Could you check a few things on this drawing? It's one solid part, dimensions in mm from its lowest x, y, z. A direction names the side the tool comes from. Round coordinates to 2 decimals unless told otherwise and drop trailing zeros. Loops run counter-clockwise (first coordinate to the right, second up) from the corner with the lowest first, then second, coordinate; pieces in that order, holes last. Notation, with made-up numbers: (29, 83.5) -> (88, 83.5) arc R34 cw to (88, 121.5) -> close; hole circle Ø10 at (56.5, -13). An arc over 180 degrees is marked (long way). Write each question's results on one line, items separated by ' | '.
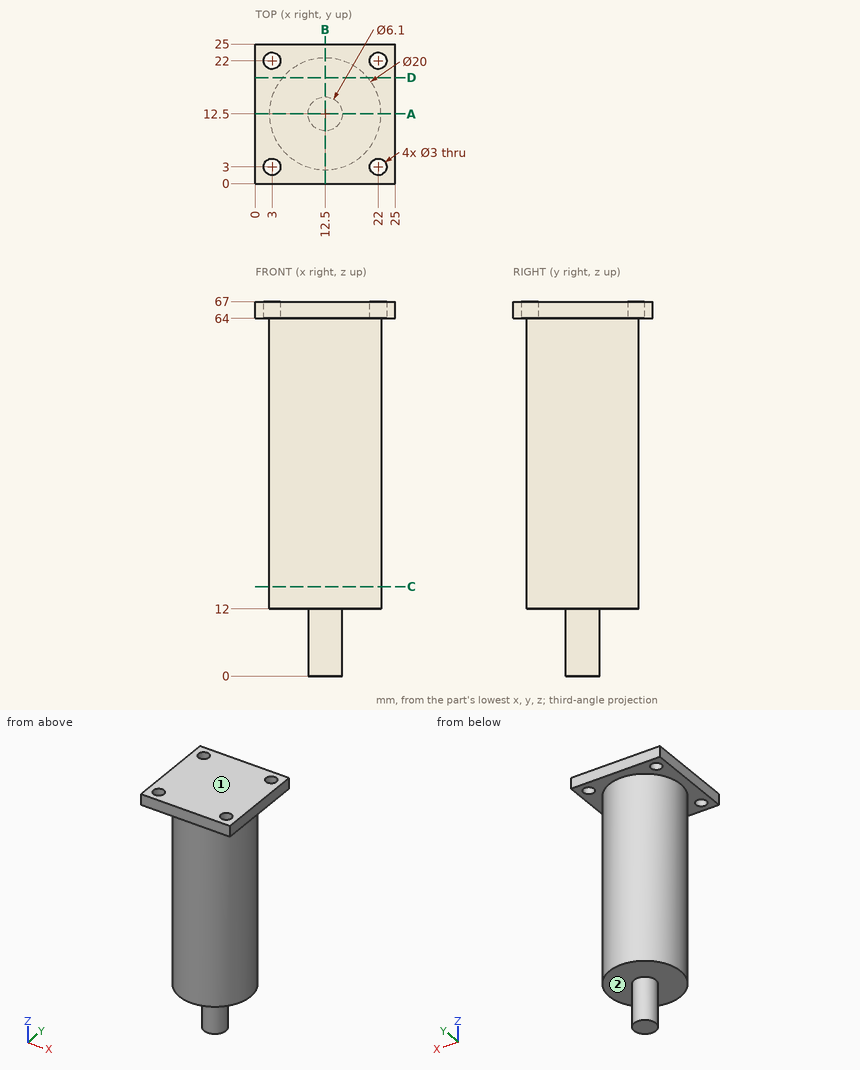
1) I want a section at D-D, the plane y = 19. Write out the boundary of the cut face in (x, z).
Model answer:
outline: (0, 64) -> (4.9, 64) -> (4.9, 12) -> (20.1, 12) -> (20.1, 64) -> (25, 64) -> (25, 67) -> (0, 67) -> close
2) I want a section at A-A, the plane y = 12.5. Write out the boundary of the cut face in (x, z), plus the area to 3 significant figures.
Model answer:
outline: (0, 64) -> (2.5, 64) -> (2.5, 12) -> (9.45, 12) -> (9.45, 0) -> (15.55, 0) -> (15.55, 12) -> (22.5, 12) -> (22.5, 64) -> (25, 64) -> (25, 67) -> (0, 67) -> close | area: 1,190 mm2
3) I want a section at C-C, the plane z = 16. Write out the boundary of the cut face in (x, y), plus the area to 3 significant figures.
Model answer:
outline: circle Ø20 at (12.5, 12.5) | area: 314 mm2
4) For the marked faces 1 and 2, which set-ups out of +Z, -Z, +X, -X, +Y, -Y let a thin tool reach every point of the face, with its end or its side?
Model answer:
face 1: +Z, +X, -X, +Y, -Y | face 2: -Z
5) I need wall thicknesses on line 1 (Y direction, x = 3, z = 64.6); line 2 (Z direction, x = 6.25, y = 17); line 3 (Z direction, x = 23, y = 6.5). Which ranges of each line are inside material? Lowest first, please.
Model answer:
line 1: y = 0 to 1.5, 4.5 to 20.5, 23.5 to 25 | line 2: z = 12 to 67 | line 3: z = 64 to 67
6) I'm going to push flat-ended pins straight in: pin 1 (2.5 mm diameter, centred on x = 3, y = 22, fed in from -Z); pin 2 (4 mm diameter, centred on x = 14, y = 21, fed in from -Z); pin 3 (4 mm diameter, centred on y = 14.5, z = 49, fed in from +X); pin 4 (10 mm diameter, centred on x = 19.5, z = 53.5, fed in from +Y). Where does each tip first touch, or does it pass through?
Model answer:
pin 1: passes through | pin 2: stops at z = 12 | pin 3: stops at x = 22.5 | pin 4: stops at y = 22.3
